The model under review builds one solid part; all positions refer to its coordinate system, in mm. A direction names the side the tool comes from. Round coordinates to 2 decimals unless told otherwise and drop trailing zeros. Write each loop counter-clockwise with the first axis right and the second up, starting at its lowest first coordinate (ties: lowest second). Pieces come first, ordered by that corner, then holes.
Item 1: Draft analysis for pull direction Y (two halves, no side actions). For faces 4 (the face through (10, 20, 0)), 5 (the face through (0, -13, -6)), 6 (the face through (10.54, 17.44, 0.28)), state which applies: +Y half, -Y half, draft (parallel to the pull), parting line (faces both ways), or undercut.
Item 2: Machinability: for faces 1 (the face through (10, -45, 0)), 2 (the face through (10, 12, -2)), 3 (the face through (10, -37, -2)), which of the approach directions +Z, -Z, +X, -X, +Y, -Y give a long, thin tool a straight path to every point of the face, cutting with its end or side? Answer none if there is none.
Item 3: Clearance check with flat-ended pins moving along their axes: pin 1 Ø7.5 at (x, y) = (6, -34.5) entering from -Z; pin 2 Ø1.5 at (x, z) = (15.5, -6.5) entering from +Y; pin 3 Ø10.5 at (x, z) = (14.5, -7.5) entering from -Y; pin 4 Ø4 at (x, y) = (10, 15) entering from -Z. State where each tip first meets the part, or that it passes through.
Item 4: Add section C-C (z = 1.25). Give the boundary of the cut face in (x, y), plus the area to 3 significant figures.
Item 5: To check wall thickness, follow L1, parallel to X at y = -40, z = 1.4; L2, parallel to Y at x = 10, z = -0.6; L3, parallel to Y at x = 10, z = 0.5. State the ranges of each line that lie inside material, in increasing order.
Item 6: Add section A-A (y = 15). Give the boundary of the cut face in (x, z), plus the area to 3 significant figures.
Item 7: Add section D-D (z = -3). Give the boundary of the cut face in (x, y).
Item 8: Add section B-B (x = 10). Give the boundary of the cut face in (y, z).
Autodesk Fusion 360 part; units mm, degrees
sketch "Boceto1" plane through (0, 0, 0) normal (1, 0, 0) x (0, 1, 0)
  line L0 (-30, 20) -> (5, 20)
  line L1 (5, 20) -> (5, -15)
  line L2 (5, -15) -> (-30, -15)
  line L3 (-30, -15) -> (-30, 20)
extrude "Extruir1" add sketch "Boceto1" along normal blind 20
sketch "Boceto2" plane through (20, 0, 0) normal (1, 0, 0) x (0, 1, 0)
  line L0 (-30, -15) -> (5, -15)
  line L1 (5, -15) -> (5, 20)
  line L2 (5, 20) -> (-30, 20)
  line L3 (-30, 20) -> (-30, -15)
  circle A0 centre (-12.543, 2.5) radius 7.5
  dimension "d3" = 15
extrude "Extruir2" cut sketch "Boceto2" against normal blind 20 contours A0
sketch "Boceto3" plane through (20, 0, 0) normal (1, 0, 0) x (0, 1, 0)
  circle A0 centre (-12.543, 2.5) radius 7.5
  line L0 (-30, -15) -> (5, -15)
  line L1 (5, -15) -> (5, 20)
  line L2 (5, 20) -> (-30, 20)
  line L3 (-30, 20) -> (-30, -15)
  line L4 (-30, 2.5) -> (5, 2.5)
  line L5 (5, 2.5) -> (5, 20)
  line L6 (5, 20) -> (-30, 20)
  line L7 (-30, 20) -> (-30, 2.5)
extrude "Extruir3" cut sketch "Boceto3" against normal blind 20 contours A0 L1 L2 L3 L4 L5 L6 L7
sketch "Boceto4" plane through (0, -30, 0) normal (0, -1, 0) x (1, 0, 0)
  line L0 (20, 2.5) -> (0, 2.5)
  line L1 (0, 2.5) -> (0, -15)
  line L2 (0, -15) -> (20, -15)
  line L3 (20, -15) -> (20, 2.5)
  line L4 (0, 2.5) -> (20, 2.5)
  line L5 (20, 2.5) -> (20, -2)
  line L6 (20, -2) -> (0, -2)
  line L7 (0, -2) -> (0, 2.5)
extrude "Extruir4" add sketch "Boceto4" along normal blind 15 contours L0 L1 L3 L4 L5 L6 L7
sketch "Boceto5" plane through (0, 5, 0) normal (0, 1, 0) x (-1, 0, 0)
  line L0 (0, 2.5) -> (-20, 2.5)
  line L1 (-20, 2.5) -> (-20, -15)
  line L2 (-20, -15) -> (0, -15)
  line L3 (0, -15) -> (0, 2.5)
sketch "Boceto6" plane through (0, 5, 0) normal (0, 1, 0) x (-1, 0, 0)
  line L0 (-20, 2.5) -> (0, 2.5)
  line L1 (0, 2.5) -> (0, -2)
  line L2 (0, -2) -> (-20, -2)
  line L3 (-20, -2) -> (-20, 2.5)
extrude "Extruir5" add sketch "Boceto6" along normal blind 15
sketch "Boceto7" plane through (0, 0, 2.5) normal (0, 0, 1) x (-1, 0, 0)
  line L0 (-20, 45) -> (-20, 20.043)
  line L1 (-20, 20.043) -> (0, 20.043)
  line L2 (0, 20.043) -> (0, 45)
  line L3 (0, 45) -> (-20, 45)
  circle A0 centre (-10, 40) radius 2.5
  circle A1 centre (-10, -15) radius 2.5
  dimension "d12" = 5
  dimension "d13" = 5
extrude "Extruir6" cut sketch "Boceto7" against normal blind 4.5 contours A0 | A1
Numbers:
1. face 4: +Y half
1. face 5: draft
1. face 6: undercut
2. face 1: +Z, -Z, +X, -X, -Y
2. face 2: -Z, +X, -X, +Y
2. face 3: -Z, +X, -X, -Y
3. pin 1: stops at z = -2
3. pin 2: stops at y = 5
3. pin 3: stops at y = -30
3. pin 4: passes through
4. outline: (0, -45) - (20, -45) - (20, -19.94) - (0, -19.94) - close; (0, -5.15) - (20, -5.15) - (20, 20) - (0, 20) - close; hole circle Ø5 at (10, -40); hole circle Ø5 at (10, 15)
4. area: 965 mm2
5. L1: x = 0 to 7.5, 12.5 to 20
5. L2: y = -45 to -42.5, -37.5 to -19.37, -5.71 to 12.5, 17.5 to 20
5. L3: y = -45 to -42.5, -37.5 to -19.77, -5.31 to 12.5, 17.5 to 20
6. outline: (0, -2) - (7.5, -2) - (7.5, 2.5) - (0, 2.5) - close; (12.5, -2) - (20, -2) - (20, 2.5) - (12.5, 2.5) - close
6. area: 67.5 mm2
7. outline: (0, -30) - (20, -30) - (20, -17.64) - (0, -17.64) - close; (0, -7.44) - (20, -7.44) - (20, 5) - (0, 5) - close
8. outline: (-45, -2) - (-42.5, -2) - (-42.5, 2.5) - (-45, 2.5) - close; (-37.5, -2) - (-30, -2) - (-30, -15) - (5, -15) - (5, -2) - (12.5, -2) - (12.5, 2.5) - (-5.04, 2.5) arc R7.5 cw to (-20.04, 2.5) - (-37.5, 2.5) - close; (17.5, -2) - (20, -2) - (20, 2.5) - (17.5, 2.5) - close
